Here's the drawing with two shaded views (mm, measured from the low corner). I have some questions. Coordinates: 2 decimals unless noted, no trailing zeros. Write each loop counter-clockwise with the first axis right and the second up, starting at its lowest first coordinate (ties: lowest second). Pieces come first, ordered by that corner, then holes. Notation, with made-up numbers: (-1, -8) -> (42, -8) arc R22 cw to (42, 5) -> close; hole circle Ø5 at (51.5, 35.5). An arc over 180 degrees is marked (long way). Use one line per item in the form item = value.
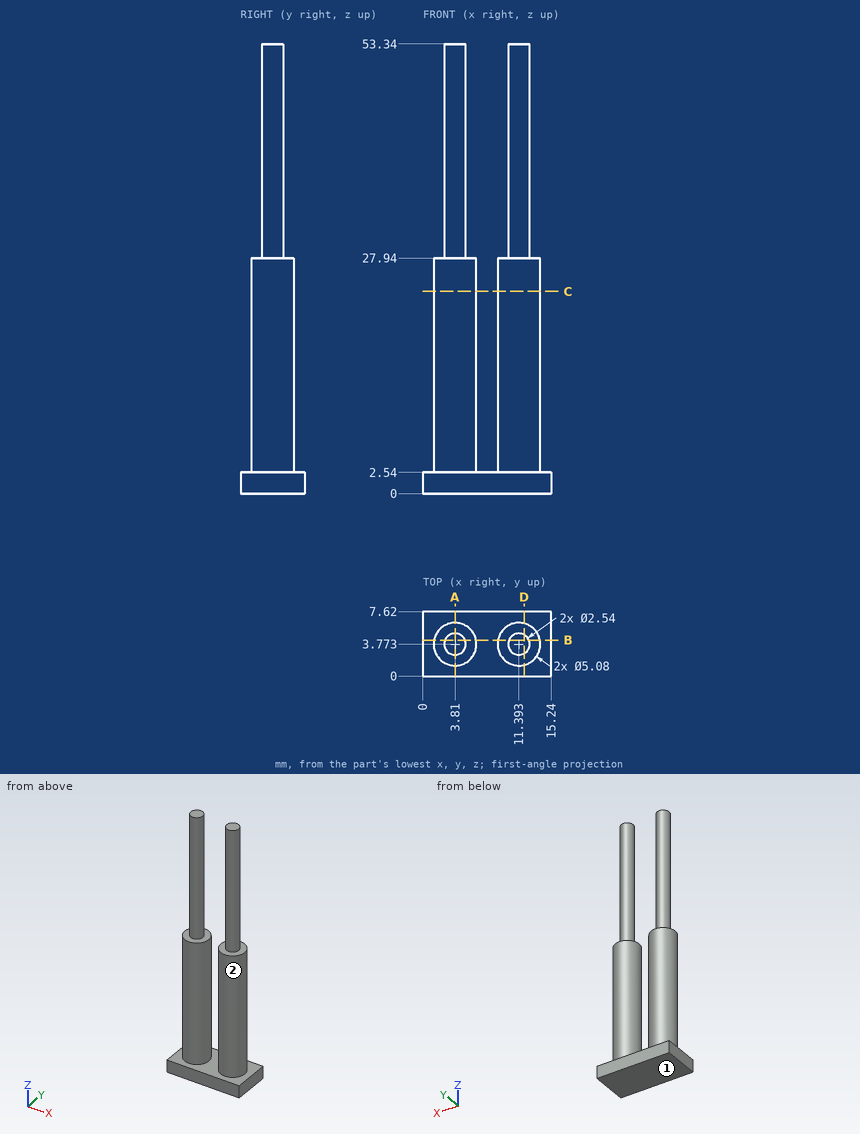
Q1. Suppose I cut it at D-D (x = 12). Write out the boundary of the cut face in (y, z).
Return value:
outline = (0, 0) -> (7.62, 0) -> (7.62, 2.54) -> (6.24, 2.54) -> (6.24, 27.94) -> (4.89, 27.94) -> (4.89, 53.34) -> (2.66, 53.34) -> (2.66, 27.94) -> (1.31, 27.94) -> (1.31, 2.54) -> (0, 2.54) -> close
Q2. Suppose I cut it at A-A (x = 3.81). Write out the boundary of the cut face in (y, z), then the cut area to 3 significant figures.
Return value:
outline = (0, 0) -> (7.62, 0) -> (7.62, 2.54) -> (6.31, 2.54) -> (6.31, 27.94) -> (5.04, 27.94) -> (5.04, 53.34) -> (2.5, 53.34) -> (2.5, 27.94) -> (1.23, 27.94) -> (1.23, 2.54) -> (0, 2.54) -> close
area = 213 mm2
Q3. Suppose I cut it at B-B (y = 4.25). Write out the boundary of the cut face in (x, z) (1 decimal).
Return value:
outline = (0, 0) -> (15.2, 0) -> (15.2, 2.5) -> (13.9, 2.5) -> (13.9, 27.9) -> (12.6, 27.9) -> (12.6, 53.3) -> (10.2, 53.3) -> (10.2, 27.9) -> (8.9, 27.9) -> (8.9, 2.5) -> (6.3, 2.5) -> (6.3, 27.9) -> (5, 27.9) -> (5, 53.3) -> (2.6, 53.3) -> (2.6, 27.9) -> (1.3, 27.9) -> (1.3, 2.5) -> (0, 2.5) -> close
Q4. If I drill on line 1 (Z direction, x = 6.5, y = 2.75); line 2 (Y direction, x = 3.75, z = 15); line 3 (X direction, y = 4, z = 28), over which ranges is the centre line in solid material (lowest first)? Write a range as from..to.
Return value:
line_1 = 0..2.54
line_2 = 1.23..6.31
line_3 = 2.56..5.06, 10.14..12.64
Q5. Will these pins go through, and if not, where does the flat tip stop? pin 1 (1 mm diameter, centred on x = 10, y = 2, fed in from -Z); pin 2 (2 mm diameter, centred on x = 10, z = 32.5, fed in from -Y) (1 decimal); pin 3 (4 mm diameter, centred on y = 4.5, z = 5.5, fed in from +X); pin 4 (3 mm diameter, centred on x = 7, z = 16, fed in from +Y).
Return value:
pin_1 = 0
pin_2 = 2.6
pin_3 = 13.93
pin_4 = 5.67
Q6. Suppose I cut it at C-C (z = 24). Write out the boundary of the cut face in (x, y).
Return value:
outline = circle Ø5.08 at (3.81, 3.77); circle Ø5.08 at (11.39, 3.77)
Q7. Thinking about a two-plate mould opening in X: for the marked faces 1 and 2, which applies, released by +X, released by -X, zero draft, split by the parting line, or undercut?
Return value:
face_1 = zero draft
face_2 = undercut
